Check sheet for the drawn part. Datum: minimum x, y, z corner. Units: mm. A direction names the side the tool comes from. Give positions to 0.01 mm unless a question says otherwise; leave off trailing zeros. Write each loop counter-clockwise with the first axis right and the second up, starting at its lowest first coordinate (ties: lowest second). Pieces come first, ordered by that corner, then holes. Notation, with made-up numbers: M -20,5.5 L -14,5.5 A28 ccw -14,32.5 Z; hole C 17.25,-19.75 d11. An arc over 180 degrees is marked long. Write item = value, one per line.
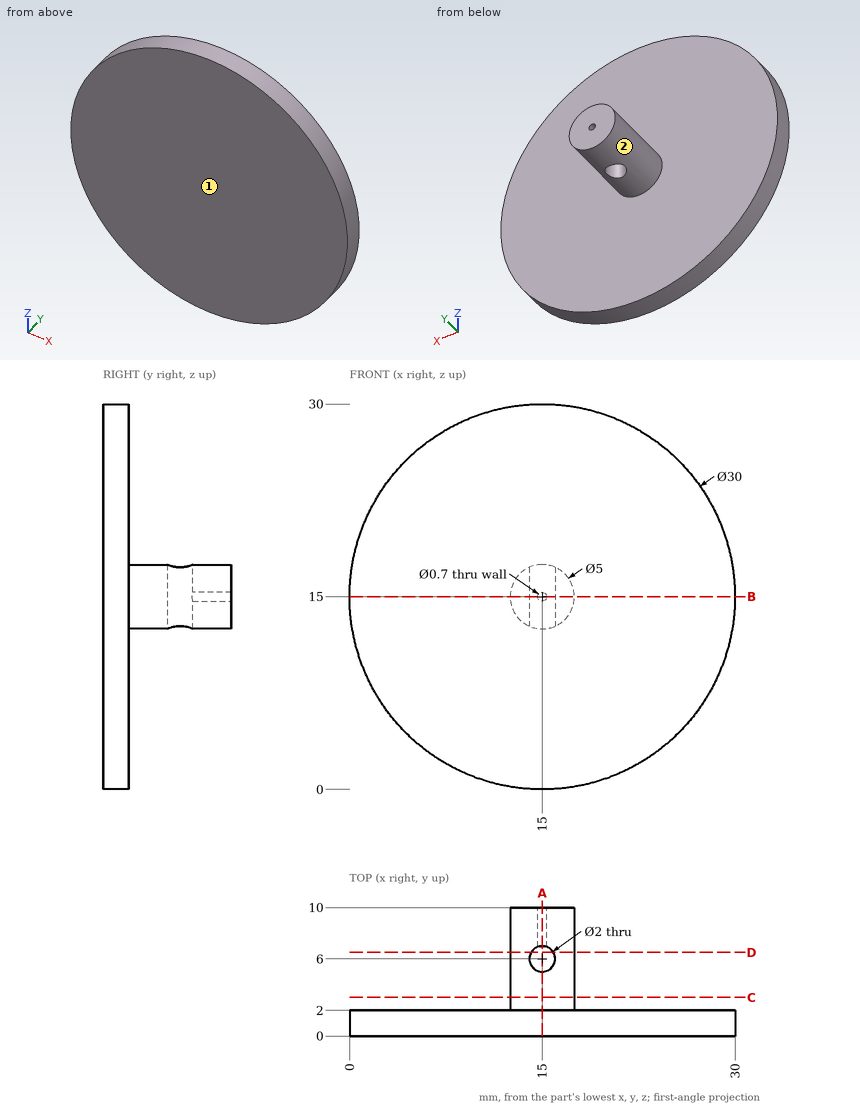
1) Tool access check on the marked faces 1 and 2. Record the directions out of +Z, -Z, +X, -X, +Y, -Y that give a thin tool (end or side, any length) a straight path to the whole face; none if there is none.
From the geometry:
face_1 = +Z, -Z, +X, -X, -Y
face_2 = +Y
2) Cross-section at C-C on y = 3. Record the boundary of the cut face in (x, z).
From the geometry:
outline = C 15,15 d5
3) Cross-section at A-A on x = 15. Record the boundary of the cut face in (y, z), plus the area to 3 significant figures.
From the geometry:
outline = M 0,0 L 2,0 L 2,12.5 L 5,12.5 L 5,17.5 L 2,17.5 L 2,30 L 0,30 Z; M 7,12.5 L 10,12.5 L 10,14.65 L 7,14.65 Z; M 7,15.35 L 10,15.35 L 10,17.5 L 7,17.5 Z
area = 87.9 mm^2
4) Cross-section at D-D on y = 6.5. Record the boundary of the cut face in (x, z).
From the geometry:
outline = M 14.13,12.65 L 14.13,17.35 A2.5 ccw Z; M 15.87,12.65 A2.5 ccw 15.87,17.35 Z
5) Depth check by flat-ended pin: P1, Ø4, axis at x = 27, y = 3, coming from the -Z side; P2, Ø3, axis at x = 18.5, z = 26.5, coming from the +Y side; P3, Ø4, axis at x = 8, z = 14, coming from the -Y side. Enter the tip coordinate at first touch or a pass-through.
From the geometry:
P1 = 4.07
P2 = 2
P3 = 0
6) Material ranges on probe 1 along X at (y, z) = (9.15, 15); probe 2 along X at (y, z) = (6, 15.1); probe 3 along Y at (x, z) = (26, 8), recorded low to high. Write a range as from..to.
From the geometry:
probe_1 = 12.5..14.65, 15.35..17.5
probe_2 = 12.5..14, 16..17.5
probe_3 = 0..2
7) Cross-section at B-B on z = 15. Record the boundary of the cut face in (x, y), plus the area to 3 significant figures.
From the geometry:
outline = M 0,0 L 30,0 L 30,2 L 17.5,2 L 17.5,10 L 15.35,10 L 15.35,6.94 A1 cw long 14.65,6.94 L 14.65,10 L 12.5,10 L 12.5,2 L 0,2 Z
area = 94.7 mm^2
